from build123d import *

# Parameters (mm, degrees)
F0_R     = 7.5
F1_DEPTH = 90
F2_R     = 4
F3_DEPTH = 10
F4_R     = 4
F5_DEPTH = 10
F6_R     = 1
F7_DEPTH = 5.0000001171
F8_DEPTH = 2
F9_R     = 1


with BuildPart() as f1:
    # F0 (on Top) → F1 (new body, symmetric)
    with BuildSketch(Plane.XY):
        Circle(F0_R)
    extrude(amount=F1_DEPTH, both=True)

    # F2 (on face) → F3 (cut)
    with BuildSketch(Plane.XY.offset(90)):
        Circle(F2_R)
    extrude(amount=-F3_DEPTH, mode=Mode.SUBTRACT)

    # F4 (on face) → F5 (cut)
    with BuildSketch(Plane(origin=(0, 0, -90), x_dir=(1, 0, 0), z_dir=(0, 0, -1))):
        Circle(F4_R)
    extrude(amount=-F5_DEPTH, mode=Mode.SUBTRACT)

    # F6 (on Front) → F7 (join, up to face)
    with BuildSketch(Plane.XZ):
        with Locations((0, 86)):
            Circle(F6_R)
        with Locations((0, -86)):
            Circle(F6_R)
    extrude(amount=F7_DEPTH)

    # F8 (cut): faces of the model
    f8_faces = [f1.faces().sort_by_distance(p)[0] for p in [
        (0, 0, 86),
        (0, 0, -86),
    ]]
    extrude(f8_faces, amount=-F8_DEPTH, mode=Mode.SUBTRACT)

    # F9
    f9_edges = [f1.edges().sort_by_distance(p)[0] for p in [
        (-7.5, 0, -90),
        (-4, 0, -90),
        (-7.5, 0, 90),
        (-4, 0, 90),
    ]]
    fillet(f9_edges, radius=F9_R)


solid = f1.part
For this review, take the finished solid that the model builds, in its own axes (mm). Round coordinates to 2 decimals unless told otherwise and drop trailing zeros. Write each loop counter-clockwise with the first axis right and the second up, starting at its lowest first coordinate (ties: lowest second). Pieces come first, ordered by that corner, then holes. Notation, with made-up numbers: (-19, -4) - (22, -4) arc R26 cw to (22, 10) - close; hole circle Ø10 at (-21, -7.75). An arc over 180 degrees is marked (long way). Use a Markdown table: item, result.
Q1. We need section B-B (z = 69). Give the boundary of the cut face in (x, y), plus the area to 3 significant figures.
Derived:
| item | result |
|---|---|
| outline | circle Ø15 at (0, 0) |
| area | 177 mm2 |
Q2. Wall thickness on line 1 along Y through (x, z) = (0, 84.25); line 2 along Z through (x, y) = (-0.5, 2.5); line 3 along X through (y, z) = (-0.5, 23): over which ranges is each line inside the solid? List them lowest first.
Derived:
| item | result |
|---|---|
| line 1 | y = -7.5 to -4, 4 to 7.5 |
| line 2 | z = -80 to 80 |
| line 3 | x = -7.48 to 7.48 |
Q3. The part is to be moulded in two halves that separate along Y. For faces 1 (the cylindrical face through (-7.493, 0.33, 1.246)), 2 (the flat face through (0, 0, -80)), 3 (the flat face through (2, -5, 90)), say which applies: pulls with the +Y half, pulls with the -Y half, needs draft (parallel to the pull), parting line crosses it, or undercut.
Derived:
| item | result |
|---|---|
| face 1 | parting line crosses it |
| face 2 | undercut |
| face 3 | needs draft |
Q4. Clearance check with flat-ended pins moving along their axes: pin 1 (6.5 mm diameter, centred on x = 0, y = 0, fed in from +Z); pin 2 (2 mm diameter, centred on y = 6, z = -58, fed in from -X); pin 3 (5 mm diameter, centred on x = 0, y = 0, fed in from -Z); pin 4 (1.6 mm diameter, centred on x = -0.5, z = -86, fed in from +Y). State where each tip first meets the part, or that it passes through.
Derived:
| item | result |
|---|---|
| pin 1 | stops at z = 87 |
| pin 2 | stops at x = -5.59 |
| pin 3 | stops at z = -87 |
| pin 4 | stops at y = 7.5 |
Q5. We need section A-A (y = 0). Give the boundary of the cut face in (x, z), plus the area to 3 significant figures.
Derived:
| item | result |
|---|---|
| outline | (-7.5, -89) arc R1 ccw to (-6.5, -90) - (-5, -90) arc R1 ccw to (-4, -89) - (-4, -80) - (4, -80) - (4, -89) arc R1 ccw to (5, -90) - (6.5, -90) arc R1 ccw to (7.5, -89) - (7.5, 89) arc R1 ccw to (6.5, 90) - (5, 90) arc R1 ccw to (4, 89) - (4, 80) - (-4, 80) - (-4, 89) arc R1 ccw to (-5, 90) - (-6.5, 90) arc R1 ccw to (-7.5, 89) - close |
| area | 2,540 mm2 |
